Part print with two shaded views. Sizes in mm from the minimum x, y, z corner. A direction names the side the tool comes from. Give positions to 0.01 mm unless a question says otherwise; leave off trailing zeros. Write each loop counter-clockwise with the first axis right and the second up, starting at its lowest first coordinate (ties: lowest second). Pieces come first, ordered by that corner, then holes. Notation, with made-up numbers: M 33,33 L 81,33 A31 ccw 81,64 Z; hole C 67.25,57.5 d2. An arc over 180 degrees is marked long. One line per item, written item: value. Start each with the question number.
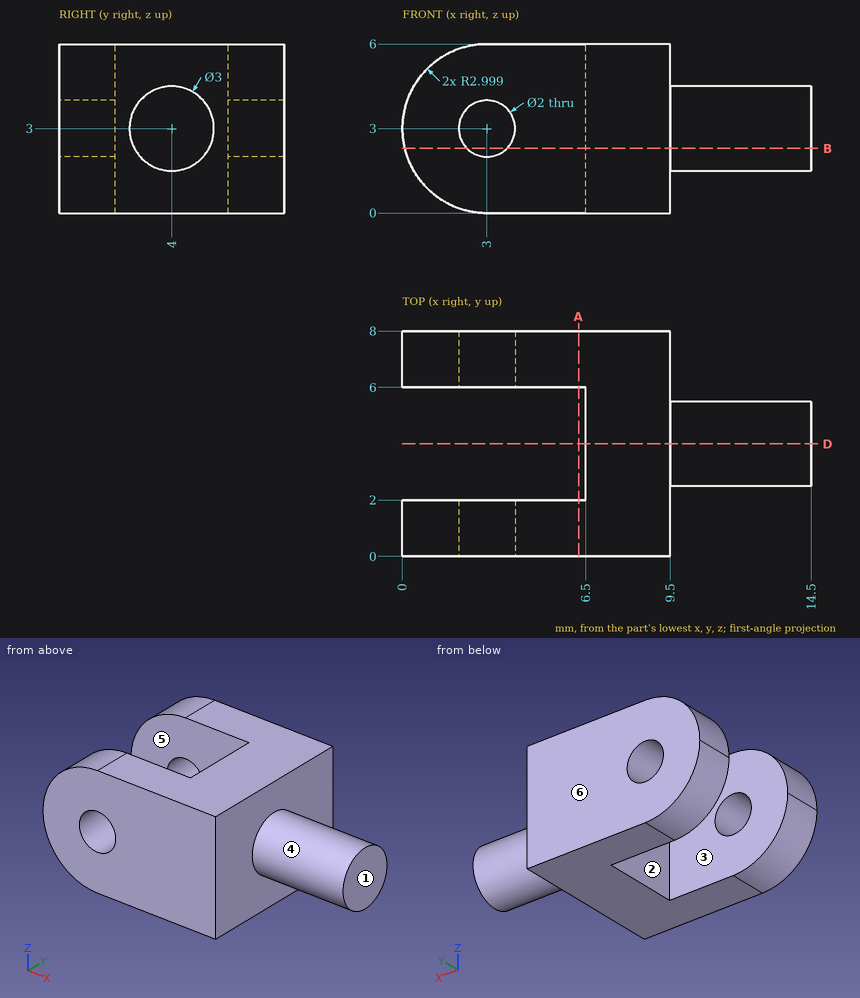
1) Band-saw the part on B-B (z = 2.3). List the corners of the cut face in (x, y) (1 decimal).
2) Mould opens along Y. For the marked faces 1, 2, 3 and 4 say: released by +Y, released by -Y, zero draft, split by the parting line, or undercut.
3) Band-saw the part on D-D (y = 4). List the corners of the cut face in (x, z), then the cut area to 3 significant figures.
4) Probe line 1 along Y through (x, z) = (2.75, 4.25); line 2 along Z through (x, y) = (3, 1.3); line 3 along X through (y, z) = (6.45, 3). List the from-to ranges inside material, lowest first. Write a range as from..to.
5) Band-saw the part on A-A (x = 6.25). List the corners of the cut face in (y, z).
6) Tool access for the marked faces 5 and 6: list every direction of +Z, -Z, +X, -X, +Y, -Y with a clear straight run to the whole face (end or side of a thin tool).
Model answer:
1. outline: M 0.1,0 L 2.3,0 L 2.3,2 L 0.1,2 Z; M 0.1,6 L 2.3,6 L 2.3,8 L 0.1,8 Z; M 3.7,0 L 9.5,0 L 9.5,2.7 L 14.5,2.7 L 14.5,5.3 L 9.5,5.3 L 9.5,8 L 3.7,8 L 3.7,6 L 6.5,6 L 6.5,2 L 3.7,2 Z
2. face 1: zero draft
2. face 2: undercut
2. face 3: undercut
2. face 4: split by the parting line
3. outline: M 6.5,0 L 9.5,0 L 9.5,1.5 L 14.5,1.5 L 14.5,4.5 L 9.5,4.5 L 9.5,6 L 6.5,6 Z
3. area: 33.0 mm²
4. line 1: y = 0..2, 6..8
4. line 2: z = 0..2, 4..6
4. line 3: x = 0..2, 4..9.5
5. outline: M 0,0 L 2,0 L 2,6 L 0,6 Z; M 6,0 L 8,0 L 8,6 L 6,6 Z
6. face 5: +Z, -Z, -X
6. face 6: +Z, -Z, +X, -X, +Y
